Design review of the part built by this model. Coordinates are the model's own, in mm. Coordinates: 2 decimals unless noted, no trailing zeros. Order: outer loops, then holes, each group sorted by start corner. A loop starts at its lowest first (then second) coordinate and runs counter-clockwise, first axis right, second up. Notation, with made-up numbers: M 12.25,83.25 L 62.25,83.25 A24 ccw 62.25,108.25 Z; hole C 62.5,51 d9. An arc over 180 degrees is marked long. Answer in a Markdown table with one row per item.
from build123d import *

# Parameters (mm, degrees)
F0_R     = 4.7625
F1_DEPTH = 12.7
F2_W     = 304.8
F2_H     = 97.490124
F2_R     = 4.7625
F3_DEPTH = 12.7


with BuildPart() as f1:
    # F0 (on Front) → F1 (new body)
    with BuildSketch(Plane.XZ):
        with BuildLine():
            ThreePointArc((-570.950153, 813.38195), (-800.269597, 644.048616), (-1078.950153, 584.062505))
            Line((-1078.950153, 584.062505), (-1078.950153, 571.362505))
            Line((-1078.950153, 571.362505), (-1739.350153, 571.362505))
            Line((-1739.350153, 571.362505), (-1739.350153, 517.387505))
            Line((-1739.350153, 517.387505), (-1739.350153, 498.337505))
            Line((-1739.350153, 498.337505), (-1739.350153, 431.662505))
            Line((-1739.350153, 431.662505), (-1078.950153, 431.662505))
            ThreePointArc((-1078.950153, 431.662505), (-840.528034, 466.655442), (-622.216208, 568.682689))
            Line((-622.216208, 568.682689), (-351.904281, 803.615156))
            ThreePointArc((-351.904281, 803.615156), (-213.788636, 868.163006), (-62.950153, 890.301394))
            ThreePointArc((-62.950153, 890.301394), (13.249847, 966.501394), (-62.950153, 1042.701394))
            ThreePointArc((-62.950153, 1042.701394), (-341.630708, 982.715283), (-570.950153, 813.38195))
        make_face()
        with Locations((-722.51368, 604.881358)):
            Circle(F0_R, mode=Mode.SUBTRACT)
        with Locations((-747.209384, 629.577062)):
            Circle(F0_R, mode=Mode.SUBTRACT)
        Polygon((-357.898706, 879.210343), (-317.464643, 909.96301), (-277.03058, 940.715678), (-269.342413, 930.607162), (-350.210539, 869.101827), align=None, mode=Mode.SUBTRACT)
    extrude(amount=F1_DEPTH)

    # F2 (on face) → F3 (join)
    with BuildSketch(Plane.XZ.offset(12.7)):
        with Locations((-1586.950153, 382.917443)):
            Rectangle(F2_W, F2_H)
        with Locations((-1612.350153, 410.372381)):
            Circle(F2_R, mode=Mode.SUBTRACT)
    extrude(amount=-F3_DEPTH)


solid = f1.part
(1) Add section A-A, the plane y = -3. Give the boundary of the cut face in (x, z) (1 decimal), and give its area (3 significant figures).
Return value:
| item | result |
|---|---|
| outline | M -1739.4,334.2 L -1434.6,334.2 L -1434.6,431.7 L -1079,431.7 A829.7 ccw -622.2,568.7 L -351.9,803.6 A524.9 cw -63,890.3 A76.2 ccw -63,1042.7 A677.3 ccw -571,813.4 A677.3 cw -1079,584.1 L -1079,571.4 L -1739.4,571.4 Z; hole C -1612.4,410.4 d9.5; hole C -747.2,629.6 d9.5; hole C -722.5,604.9 d9.5; hole M -357.9,879.2 L -350.2,869.1 L -269.3,930.6 L -277,940.7 Z |
| area | 304,000 mm2 |
(2) Add section B-B, the plane x = -1097. Give the boundary of the cut face in (y, z).
Return value:
| item | result |
|---|---|
| outline | M -12.7,431.66 L 0,431.66 L 0,571.36 L -12.7,571.36 Z |
(3) Add section C-C, the plane z = 536.5. Give the boundary of the cut face in (x, y), and give its area (3 significant figures).
Return value:
| item | result |
|---|---|
| outline | M -1739.35,-12.7 L -675.24,-12.7 L -675.24,0 L -1739.35,0 Z |
| area | 13,500 mm2 |
(4) For line 1 along Z through (x, y) = (-1156.5, -7); line 2 along Z through (x, y) = (-1530.5, -4); line 3 along X through (y, z) = (-9.75, 530.5), list the stretches that pass through material, from the lowest coordinate up. Write a range as from..to.
Return value:
| item | result |
|---|---|
| line 1 | z = 431.66..571.36 |
| line 2 | z = 334.17..571.36 |
| line 3 | x = -1739.35..-686.21 |
(5) Insertion check: pin 1 Ø3 at (y, z) = (-11.5, 805.5) entering from +X; pin 2 Ø4 at (x, y) = (-1262, -9.5) entering from +Z; pin 3 Ø12.5 at (x, z) = (-1612.35, 410.37) entering from -Y; pin 4 Ø3 at (y, z) = (-9, 825.5) entering from -X. Each pin has a flat end and moves straight along its axis. Give the tip position at first contact, or say it passes through.
Return value:
| item | result |
|---|---|
| pin 1 | stops at x = -346.7 |
| pin 2 | stops at z = 571.36 |
| pin 3 | stops at y = -12.7 |
| pin 4 | stops at x = -561.38 |
(6) Draft analysis for pull direction Z (two halves, no side actions). For faces 1 (the flat face through (-867, 0, 611)), 2 (the flat face through (-488.952, -6.261, 684.504)), 3 (the cylindrical face through (13.23, -6.26, 964.83)), 4 (the flat face through (-309.21, -6.261, 900.285)), state which applies: pulls with the +Z half, pulls with the -Z half, needs draft (parallel to the pull), parting line crosses it, or undercut.
Return value:
| item | result |
|---|---|
| face 1 | needs draft |
| face 2 | pulls with the -Z half |
| face 3 | parting line crosses it |
| face 4 | undercut |
